from build123d import *

# Parameters (mm, degrees)
SKETCH1_W           = 103
SKETCH1_H           = 73
BOSS_EXTRUDE1_DEPTH = 2
SKETCH2_W           = 95
SKETCH2_H           = 65
BOSS_EXTRUDE2_DEPTH = 5
BOSS_EXTRUDE3_DEPTH = 2
SKETCH12_W          = 2.8
SKETCH12_H          = 3.5
CUT_EXTRUDE3_DEPTH  = 7
CUT_EXTRUDE3_TAPER  = -66
FILLET4_R           = 4
CUT_EXTRUDE5_DEPTH  = 5
FILLET5_R           = 2
FILLET6_R           = 5


with BuildPart() as part:
    # Sketch1 → Boss-Extrude1 (new body)
    with BuildSketch(Plane(origin=(0, 0, 0), x_dir=(1, 0, 0), z_dir=(0, 1, 0))):
        Rectangle(SKETCH1_W, SKETCH1_H)
    extrude(amount=BOSS_EXTRUDE1_DEPTH)

    # Sketch2 → Boss-Extrude2 (add)
    with BuildSketch(Plane.XZ):
        Rectangle(SKETCH2_W, SKETCH2_H)
    extrude(amount=BOSS_EXTRUDE2_DEPTH)

    # Sketch3 → Boss-Extrude3 (add)
    with BuildSketch(Plane(origin=(0, 2, 0), x_dir=(1, 0, 0), z_dir=(0, 1, 0))):
        with BuildLine():
            Line((-7, -36.5), (7, -36.5))
            ThreePointArc((7, -36.5), (0, -43.5), (-7, -36.5))
        make_face()
    boss_extrude3 = extrude(amount=-BOSS_EXTRUDE3_DEPTH)

    # Mirror1: Boss-Extrude3 across plane
    add(boss_extrude3.mirror(Plane.XY))

    # Sketch12 → Cut-Extrude3 (cut)
    with BuildSketch(Plane.XZ.offset(5)):
        with Locations((28.702273545, 0.998760933)):
            Rectangle(SKETCH12_W, SKETCH12_H)
    extrude(amount=-CUT_EXTRUDE3_DEPTH, taper=CUT_EXTRUDE3_TAPER, mode=Mode.SUBTRACT)

    # Fillet4
    fillet4_edges = [part.edges().sort_by_distance(p)[0] for p in [
        (51.5, 1, 36.5),
        (-51.5, 1, 36.5),
        (-51.5, 1, -36.5),
        (51.5, 1, -36.5),
    ]]
    fillet(fillet4_edges, radius=FILLET4_R)

    # Sketch13 → Cut-Extrude5 (cut)
    with BuildSketch(Plane.XZ.offset(5)):
        with BuildLine():
            ThreePointArc((-9.102862796, -4.001239067), (-14.007432374, -8.905808645), (-9.102862796, -13.810378223))
            Line((-9.102862796, -13.810378223), (15.897137204, -13.810378223))
            Line((15.897137204, -13.810378223), (15.897137204, -23.810378223))
            Line((15.897137204, -23.810378223), (-9.102862796, -23.810378223))
            ThreePointArc((-9.102862796, -23.810378223), (-24.007432374, -8.905808645), (-9.102862796, 5.998760933))
            Line((-9.102862796, 5.998760933), (10.507409885, 5.998760933))
            Line((10.507409885, 5.998760933), (15.897137204, 5.998760933))
            Line((15.897137204, 5.998760933), (15.897137204, -4.001239067))
            Line((15.897137204, -4.001239067), (14.523166563, -4.001239067))
            Line((14.523166563, -4.001239067), (-9.102862796, -4.001239067))
        make_face()
    extrude(amount=-CUT_EXTRUDE5_DEPTH, mode=Mode.SUBTRACT)

    # Fillet5
    fillet5_edges = [part.edges().sort_by_distance(p)[0] for p in [
        (15.897137204, 0, -18.810378223),
        (15.897137204, 0, 0.998760933),
        (15.897137204, -5, -18.810378223),
        (15.897137204, -5, 0.998760933),
    ]]
    fillet(fillet5_edges, radius=FILLET5_R)

    # Fillet6
    fillet6_edges = [part.edges().sort_by_distance(p)[0] for p in [
        (-47.5, -2.5, -32.5),
        (47.5, -2.5, -32.5),
        (47.5, -2.5, 32.5),
        (-47.5, -2.5, 32.5),
    ]]
    fillet(fillet6_edges, radius=FILLET6_R)


solid = part.part
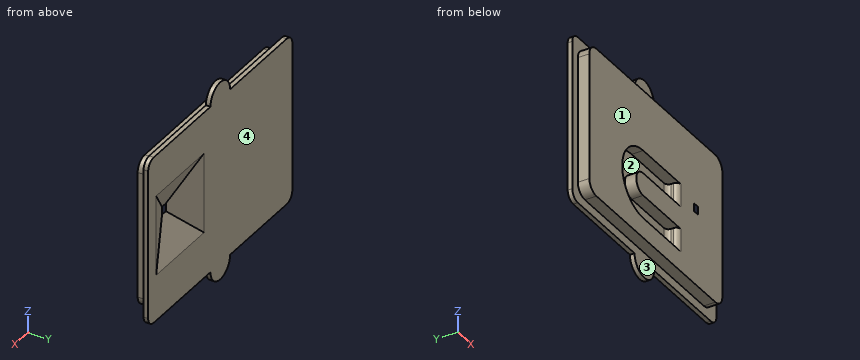
Verification items for the finished model (mm, model axes). Face numbers are marked on the shaded views. A direction names the side the tool comes from. Round coordinates to 2 decimals unless told otherwise and drop trailing zeros. Loops run counter-clockwise (first coordinate to the right, second up) from the corner with the lowest first, then second, coordinate; pieces in that order, holes last. Notation, with made-up numbers: (52.25, 76) - (99.25, 76) arc R24 ccw to (99.25, 88) - close; hole circle Ø3 at (-27, 27). An arc over 180 degrees is marked (long way). Answer in a Markdown table with one row per item. Add a question column.
Q1. Tool access check on the marked faces 3 and 4. Record the directions out of +Z, -Z, +X, -X, +Y, -Y that give a thin tool (end or side, any length) a straight path to the whole face; none if there is none.
Q2. Section check D-D on z = -38. Enter the section's corners in (x, y).
Q3. Release check for a two-part mould opening along Z. For the marked faces 1 and 2 record: pulls with the +Z half, pulls with the -Z half, needs draft (parallel to the pull), parting line crosses it, or undercut.
Q4. Section check B-B on z = -18. Enter the section's corners in (x, y).
Q5. Section check C-C on x = -37.5. Enter the section's corners in (y, z).
Q6. Section check A-A on x = 0. Enter the section's corners in (y, z).
Q7. Gauge pin test, flat ends, axial feed: pin 1 (2 mm diameter, centred on x = -20.5, y = 1.5, fed in from +Z); pin 2 (2.5 mm diameter, centred on x = 3, y = -2, fed in from +Z); pin 3 (1.5 mm diameter, centred on y = -3, z = 19, fed in from +X). Record the tip position at first contact, or that the pin passes through.
Q8. Material ranges on line 1 (Z direction, x = 10, y = -2.75); line 2 (Z direction, x = 37, y = -1.25); line 3 (X direction, y = -3, z = -22), recorded low to high.
Found:
| question | item | result |
|---|---|---|
| 1 | face 3 | -Y |
| 1 | face 4 | +Z, -Z, +X, -X, +Y |
| 2 | outline | (-6.84, 0) - (6.84, 0) - (6.84, 2) - (-6.84, 2) - close |
| 3 | face 1 | needs draft |
| 3 | face 2 | undercut |
| 4 | outline | (-51.5, 0) - (-47.5, 0) - (-47.5, -5) - (-20.91, -5) - (-20.91, 0) - (13.9, 0) arc R2 cw to (15.9, -2) - (15.9, -3) arc R2 ccw to (17.9, -5) - (47.5, -5) - (47.5, 0) - (51.5, 0) - (51.5, 2) - (-51.5, 2) - close |
| 5 | outline | (-5, -32.5) - (0, -32.5) - (0, -36.5) - (2, -36.5) - (2, 36.5) - (0, 36.5) - (0, 32.5) - (-5, 32.5) - close |
| 6 | outline | (-5, -32.5) - (0, -32.5) - (0, -43.5) - (2, -43.5) - (2, 43.5) - (0, 43.5) - (0, 32.5) - (-5, 32.5) - (-5, 6) - (0, 6) - (0, -4) - (-5, -4) - (-5, -13.81) - (0, -13.81) - (0, -23.81) - (-5, -23.81) - close |
| 7 | pin 1 | stops at z = 36.5 |
| 7 | pin 2 | stops at z = 32.5 |
| 7 | pin 3 | stops at x = 47.5 |
| 8 | line 1 | z = -32.5 to -23.81, -13.81 to -4, 6 to 32.5 |
| 8 | line 2 | z = -32.5 to -9.17, 11.17 to 32.5 |
| 8 | line 3 | x = -47.5 to -16.22, 15.9 to 47.5 |
